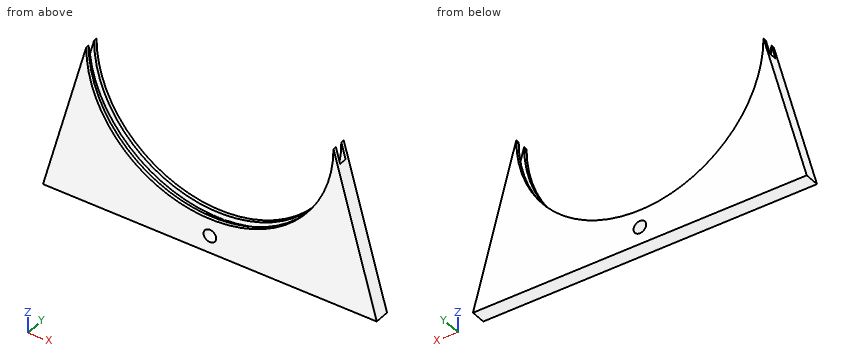
```python
from build123d import *

# Parameters (mm, degrees)
SKETCH005_R     = 2.55
PAD003_DEPTH    = 3
SKETCH006_R     = 52.1
POCKET_DEPTH    = 1.6
SKETCH011_W     = 8.2
SKETCH011_H     = 9
POCKET003_DEPTH = 1.55


with BuildPart() as part:
    # Sketch005 → Pad003 (new body, symmetric)
    with BuildSketch(Plane.XZ):
        with BuildLine():
            Line((-67.5, -64), (-50, 0))
            ThreePointArc((-50, 0), (0, -50), (50, 0))
            Line((67.5, -64), (50, 0))
            Line((-67.5, -64), (67.5, -64))
        make_face()
        with Locations((0, -57)):
            Circle(SKETCH005_R, mode=Mode.SUBTRACT)
    extrude(amount=PAD003_DEPTH, both=True)

    # Sketch006 → Pocket (cut, symmetric)
    with BuildSketch(Plane.XZ):
        Circle(SKETCH006_R)
    extrude(amount=POCKET_DEPTH, both=True, mode=Mode.SUBTRACT)

    # Sketch011 → Pocket003 (cut, symmetric)
    with BuildSketch(Plane.XZ):
        with Locations((0, -49.1)):
            Rectangle(SKETCH011_W, SKETCH011_H)
    extrude(amount=POCKET003_DEPTH, both=True, mode=Mode.SUBTRACT)


solid = part.part
```
Geometry check sheet. Reference: the model listing, model coordinates, mm. Round coordinates to 2 decimals unless told otherwise and drop trailing zeros. Order: outer loops, then holes, each group sorted by start corner. A loop starts at its lowest first (then second) coordinate and runs counter-clockwise, first axis right, second up. Notation, with made-up numbers: M 7,68.25 L 66,68.25 A13 ccw 66,84.25 Z; hole C -10,61.25 d7. An arc over 180 degrees is marked long. Answer as CSV lines item,"result".
1) Sectioned sample at D-D on z = -57. Record the cut outline in (x, y).
Entries:
outline,"M -65.59,-3 L -2.55,-3 L -2.55,3 L -65.59,3 Z; M 2.55,-3 L 65.59,-3 L 65.59,3 L 2.55,3 Z"
2) Sectioned sample at C-C on x = -15. Record the cut outline in (y, z).
Entries:
outline,"M -3,-64 L 3,-64 L 3,-47.7 L 1.6,-47.7 L 1.6,-49.89 L -1.6,-49.89 L -1.6,-47.7 L -3,-47.7 Z"
3) Sectioned sample at B-B on z = -42. Record the cut outline in (x, y).
Entries:
outline,"M -61.48,-3 L -27.13,-3 L -27.13,-1.6 L -30.83,-1.6 L -30.83,1.6 L -27.13,1.6 L -27.13,3 L -61.48,3 Z; M 27.13,-3 L 61.48,-3 L 61.48,3 L 27.13,3 L 27.13,1.6 L 30.83,1.6 L 30.83,-1.6 L 27.13,-1.6 Z"
4) Thickness scan on probe 1 along Y at (x, z) = (-5.5, -51); probe 2 along Z at (x, y) = (0, 0.15); probe 3 along X at (y, z) = (1.9, -36). Record the ranges inside material, lowest first. Write a range as [from, to].
Entries:
probe 1,"[-3, -1.6], [1.6, 3]"
probe 2,"[-64, -59.55], [-54.45, -53.6]"
probe 3,"[-59.84, -34.7], [34.7, 59.84]"
5) Gauge pin test, flat ends, axial feed: pin 1 Ø1.3 at (y, z) = (0.5, -53) entering from -X; pin 2 Ø3.5 at (x, y) = (0, 0.5) entering from +Z; pin 3 Ø2 at (y, z) = (1.5, -11.5) entering from +X. Record the tip position at first contact, or that the pin passes through.
Entries:
pin 1,"x = -64.67"
pin 2,"z = -49.98"
pin 3,"x = 53.42"
6) Sectioned sample at A-A on x = 0. Record the cut outline in (y, z).
Entries:
outline,"M -3,-64 L 3,-64 L 3,-59.55 L -3,-59.55 Z; M -3,-54.45 L 3,-54.45 L 3,-50 L 1.6,-50 L 1.6,-52.1 L 1.55,-52.1 L 1.55,-53.6 L -1.55,-53.6 L -1.55,-52.1 L -1.6,-52.1 L -1.6,-50 L -3,-50 Z"
